from build123d import *

# Parameters (mm, degrees)
F0_R     = 3.175
F1_DEPTH = 25.4


# Not quite as in the source:
# - ends of sketch curves that miss each other by under 0.0002 mm in the source are joined


with BuildPart() as f1:
    # F0 (on Front) → F1 (new body)
    with BuildSketch(Plane.XZ):
        with BuildLine():
            add(Edge.make_bspline(
                [(-228.6, 0), (-228.603328408, -20.9998549914), (-216.1362353399, -33.3187275092), (-190.5048638582, -40.5451878905)],
                knots=[0, 0, 0, 0, 96.8546122477, 96.8546122477, 96.8546122477, 96.8546122477], degree=3))
            add(Edge.make_bspline(
                [(-228.6, 0), (-228.603328408, 20.9998549914), (-216.1362353399, 33.3187275092), (-190.5048638582, 40.5451878905)],
                knots=[0, 0, 0, 0, 96.8546122477, 96.8546122477, 96.8546122477, 96.8546122477], degree=3))
            add(Edge.make_bspline(
                [(-190.5048638582, 40.5451878905), (-188.6690340196, 41.0627782819), (-186.7656708429, 41.5542443707), (-184.7945193799, 42.0209047272)],
                knots=[96.8546122477, 96.8546122477, 96.8546122477, 96.8546122477, 103.7917590678, 103.7917590678, 103.7917590678, 103.7917590678], degree=3))
            add(Edge.make_bspline(
                [(-181.8914412177, 82.4957251162), (-177.7740978469, 82.7671917451), (-166.6388871368, 81.1057466034), (-160.4841015231, 50.6684396177), (-176.6492852244, 44.2605429862), (-184.7945193799, 42.0209047272)],
                knots=[0.1201664208, 0.1201664208, 0.1201664208, 0.1201664208, 0.2987042421, 0.6454715168, 0.9336630859, 0.9336630859, 0.9336630859, 0.9336630859], degree=3))
            add(Edge.make_bspline(
                [(-190.5065755272, 81.190021553), (-187.6562706797, 81.6501805926), (-184.7832793111, 82.0849710788), (-181.8914412177, 82.4957251162)],
                knots=[152.2718692701, 152.2718692701, 152.2718692701, 152.2718692701, 159.2026765547, 159.2026765547, 159.2026765547, 159.2026765547], degree=3))
            add(Edge.make_bspline(
                [(-304.7999998765, 0.0020627141), (-304.7970834826, 48.7263819663), (-253.1268418931, 71.0804777771), (-190.5065755272, 81.190021553)],
                knots=[0.0042973705, 0.0042973705, 0.0042973705, 0.0042973705, 152.2718692701, 152.2718692701, 152.2718692701, 152.2718692701], degree=3))
            add(Edge.make_bspline(
                [(-304.8, -0.0020627142), (-304.8, -0.0006875504), (-304.7999999588, 0.0006875924), (-304.7999998765, 0.0020627141)],
                knots=[0, 0, 0, 0, 0.0042973705, 0.0042973705, 0.0042973705, 0.0042973705], degree=3))
            add(Edge.make_bspline(
                [(-304.8, -0.0020627142), (-304.7970834826, -48.7263819663), (-253.1268418931, -71.0804777771), (-190.5065755272, -81.190021553)],
                knots=[0.0042973705, 0.0042973705, 0.0042973705, 0.0042973705, 152.2718692701, 152.2718692701, 152.2718692701, 152.2718692701], degree=3))
            add(Edge.make_bspline(
                [(-190.5065755272, -81.190021553), (-187.6562706797, -81.6501805926), (-184.7832793111, -82.0849710788), (-181.8914412177, -82.4957251162)],
                knots=[152.2718692701, 152.2718692701, 152.2718692701, 152.2718692701, 159.2026765547, 159.2026765547, 159.2026765547, 159.2026765547], degree=3))
            add(Edge.make_bspline(
                [(-181.8914412177, -82.4957251162), (-177.7740978469, -82.7671917451), (-166.6388871368, -81.1057466034), (-160.4841015231, -50.6684396177), (-176.6492852244, -44.2605429862), (-184.7945193799, -42.0209047272)],
                knots=[0.1201664208, 0.1201664208, 0.1201664208, 0.1201664208, 0.2987042421, 0.6454715168, 0.9336630859, 0.9336630859, 0.9336630859, 0.9336630859], degree=3))
            add(Edge.make_bspline(
                [(-190.5048638582, -40.5451878905), (-188.6690340196, -41.0627782819), (-186.7656708429, -41.5542443707), (-184.7945193799, -42.0209047272)],
                knots=[96.8546122477, 96.8546122477, 96.8546122477, 96.8546122477, 103.7917590678, 103.7917590678, 103.7917590678, 103.7917590678], degree=3))
        make_face()
        with Locations((-228.6080516329, -50.8)):
            Circle(F0_R, mode=Mode.SUBTRACT)
        with Locations((-266.7, 0)):
            Circle(F0_R, mode=Mode.SUBTRACT)
        with Locations((-228.6080516329, 50.8)):
            Circle(F0_R, mode=Mode.SUBTRACT)
        with BuildLine():
            add(Edge.make_bspline(
                [(-190.5048638582, 40.5451878905), (-188.6690340196, 41.0627782819), (-186.7656708429, 41.5542443707), (-184.7945193799, 42.0209047272)],
                knots=[96.8546122477, 96.8546122477, 96.8546122477, 96.8546122477, 103.7917590678, 103.7917590678, 103.7917590678, 103.7917590678], degree=3))
            add(Edge.make_bspline(
                [(-184.7945193799, 42.0209047272), (-186.6694170397, 41.5053771867), (-188.587140449, 41.0252825386), (-190.5048638582, 40.5451878905)],
                knots=[0.9336630859, 0.9336630859, 0.9336630859, 0.9336630859, 1, 1, 1, 1], degree=3))
        make_face()
        with BuildLine():
            add(Edge.make_bspline(
                [(-184.7945193799, -42.0209047272), (-186.6694170397, -41.5053771867), (-188.587140449, -41.0252825386), (-190.5048638582, -40.5451878905)],
                knots=[0.9336630859, 0.9336630859, 0.9336630859, 0.9336630859, 1, 1, 1, 1], degree=3))
            add(Edge.make_bspline(
                [(-190.5048638582, -40.5451878905), (-188.6690340196, -41.0627782819), (-186.7656708429, -41.5542443707), (-184.7945193799, -42.0209047272)],
                knots=[96.8546122477, 96.8546122477, 96.8546122477, 96.8546122477, 103.7917590678, 103.7917590678, 103.7917590678, 103.7917590678], degree=3))
        make_face()
        with BuildLine():
            add(Edge.make_bspline(
                [(-190.5065755272, 81.190021553), (-187.6562706797, 81.6501805926), (-184.7832793111, 82.0849710788), (-181.8914412177, 82.4957251162)],
                knots=[152.2718692701, 152.2718692701, 152.2718692701, 152.2718692701, 159.2026765547, 159.2026765547, 159.2026765547, 159.2026765547], degree=3))
            add(Edge.make_bspline(
                [(-190.5065755272, 81.190021553), (-187.58461511, 81.7515168563), (-184.6626546928, 82.3130121597), (-181.8914412177, 82.4957251162)],
                knots=[0, 0, 0, 0, 0.1201664208, 0.1201664208, 0.1201664208, 0.1201664208], degree=3))
        make_face()
        with BuildLine():
            add(Edge.make_bspline(
                [(-190.5065755272, -81.190021553), (-187.58461511, -81.7515168563), (-184.6626546928, -82.3130121597), (-181.8914412177, -82.4957251162)],
                knots=[0, 0, 0, 0, 0.1201664208, 0.1201664208, 0.1201664208, 0.1201664208], degree=3))
            add(Edge.make_bspline(
                [(-190.5065755272, -81.190021553), (-187.6562706797, -81.6501805926), (-184.7832793111, -82.0849710788), (-181.8914412177, -82.4957251162)],
                knots=[152.2718692701, 152.2718692701, 152.2718692701, 152.2718692701, 159.2026765547, 159.2026765547, 159.2026765547, 159.2026765547], degree=3))
        make_face()
    extrude(amount=F1_DEPTH)


solid = f1.part
CAD build for the part. Positions are in the model's coordinates, mm. Coordinates: 2 decimals unless noted, no trailing zeros. Write item = value, one per line. Start each with the question number.
Q1. Cut at A-A, the plane y = -21.25. Give the number of separate pieces and of enclosed holes in the cut face, then the cut area to 3 significant figures.
Q2. Flat gauge pins, fed straight in: pin 1 Ø1 at (y, z) = (-7, -8.5) entering from -X; pin 2 Ø6 at (x, y) = (-260.5, -11.5) entering from -Z; pin 3 Ø1 at (y, z) = (-16, 53.5) entering from +X; pin 4 Ø5.5 at (x, z) = (-228.61, -50.8) entering from -Y. Where does each tip first touch, or does it go through?
Q3. Drill centre lines: L1, parallel to X at y = -15, z = -53; L2, parallel to Z at x = -193.5, y = -24; L3, parallel to Z at x = -215, y = -4.25. Where is each one in solid material? Low to high.
Q4. Pull direction Z, two halves, no side cores. Call faces 1 (the flat face through (-232, 0, 1)), 2 (the cylindrical face through (-269.22, -12.52, -1.93)): pulls with the +Z half, pulls with the -Z half, needs draft (parallel to the pull), parting line crosses it, or undercut.
Computed:
q1.separate_pieces = 1
q1.enclosed_holes = 3
q1.area = 13,400 mm²
q2.pin_1 = -304.31
q2.pin_2 = -62.41
q2.pin_3 = -166.14
q2.pin_4 = through
q3.L1 = -274.33 to -230.9, -226.32 to -166.62
q3.L2 = -80.7 to -39.66, 39.66 to 80.7
q3.L3 = -76.43 to -29.19, 29.19 to 76.43
q4.face_1 = needs draft
q4.face_2 = undercut
